from build123d import *

# Parameters (mm, degrees)
F0_R     = 2.3
F0_R_2   = 1.6
F1_DEPTH = 3
F0_R_3   = 3.05
F2_DEPTH = 2
F3_R     = 0.3
F4_SIZE  = 1


with BuildPart() as f1:
    # F0 (on Top) → F1 (new body)
    with BuildSketch(Plane.XY):
        Circle(F0_R)
        Circle(F0_R_2, mode=Mode.SUBTRACT)
    extrude(amount=F1_DEPTH)

    # F0 (on Top) → F2 (join)
    with BuildSketch(Plane.XY):
        Circle(F0_R_3)
        Circle(F0_R, mode=Mode.SUBTRACT)
    extrude(amount=F2_DEPTH)

    # F3
    f3_edges = [f1.edges().sort_by_distance(p)[0] for p in [
        (-3.05, 0, 2),
    ]]
    fillet(f3_edges, radius=F3_R)

    # F4
    f4_edges = [f1.edges().sort_by_distance(p)[0] for p in [
        (-1.6, 0, 0),
    ]]
    chamfer(f4_edges, length=F4_SIZE)


solid = f1.part
Build history of the part. All positions in model axes, mm. Round coordinates to 2 decimals unless told otherwise and drop trailing zeros. Write each loop counter-clockwise with the first axis right and the second up, starting at its lowest first coordinate (ties: lowest second). Pieces come first, ordered by that corner, then holes. Notation, with made-up numbers: (19.25, 10) - (72.25, 10) arc R26 ccw to (72.25, 34) - close; hole circle Ø9 at (32, -31). An arc over 180 degrees is marked (long way). One line per question, with ' | ' between items.
1. Drill centre lines: line 1 along Y through (x, z) = (0, 2.3); line 2 along X through (y, z) = (0.75, 0.2); line 3 along X through (y, z) = (-1, 1.65). Where is each one in solid material? Low to high. Write a range as from..to.
Results are:
line 1: -2.3..-1.6, 1.6..2.3 | line 2: -2.96..-2.28, 2.28..2.96 | line 3: -2.88..-1.25, 1.25..2.88
2. Band-saw the part on D-D, the plane z = 0.9. Write the cut outline in (x, y).
Results are:
outline: circle Ø6.1 at (0, 0); hole circle Ø3.4 at (0, 0)
3. Band-saw the part on C-C, the plane z = 1.6. Write the cut outline in (x, y).
Results are:
outline: circle Ø6.1 at (0, 0); hole circle Ø3.2 at (0, 0)
4. Mould opens along X. For faces 1 (the face through (-1.27, -0.97, 1.99)), 2 (the face through (-3.047, 0.134, 0.838)), 3 (the face through (-2, 0, 3)) say: released by +X, released by -X, zero draft, split by the parting line, or undercut.
Results are:
face 1: undercut | face 2: split by the parting line | face 3: zero draft
5. Band-saw the part on A-A, the plane y = 0. Write the cut outline in (x, z), and give its area (3 significant figures).
Results are:
outline: (-3.05, 0) - (-2.6, 0) - (-1.6, 1) - (-1.6, 3) - (-2.3, 3) - (-2.3, 2) - (-2.75, 2) arc R0.3 ccw to (-3.05, 1.7) - close; (1.6, 1) - (2.6, 0) - (3.05, 0) - (3.05, 1.7) arc R0.3 ccw to (2.75, 2) - (2.3, 2) - (2.3, 3) - (1.6, 3) - close | area: 6.16 mm^2
